from build123d import *

# Parameters (mm, degrees)
SKETCH1_R           = 1.5
BOSS_EXTRUDE1_DEPTH = 2
FILLET1_R           = 0.5
SKETCH3_R           = 2
SKETCH3_R_2         = 1.5
BOSS_EXTRUDE2_DEPTH = 0.5
BOSS_EXTRUDE2_TAPER = 5
FILLET2_R           = 0.1


with BuildPart() as part:
    # Sketch1 → Boss-Extrude1 (new body)
    with BuildSketch(Plane.XY):
        with BuildLine():
            Line((2.753751395, -0.013659805), (1.795799026, 2.087687523))
            ThreePointArc((1.795799026, 2.087687523), (1.631145222, 2.287378341), (1.388705435, 2.377988761))
            Line((1.388705435, 2.377988761), (-0.910090917, 2.599051338))
            ThreePointArc((-0.910090917, 2.599051338), (-1.165355141, 2.55630237), (-1.365045959, 2.391648566))
            Line((-1.365045959, 2.391648566), (-2.705889943, 0.511363815))
            ThreePointArc((-2.705889943, 0.511363815), (-2.796500362, 0.268924029), (-2.753751395, 0.013659805))
            Line((-2.753751395, 0.013659805), (-1.795799026, -2.087687523))
            ThreePointArc((-1.795799026, -2.087687523), (-1.631145222, -2.287378341), (-1.388705435, -2.377988761))
            Line((-1.388705435, -2.377988761), (0.910090917, -2.599051338))
            ThreePointArc((0.910090917, -2.599051338), (1.165355141, -2.55630237), (1.365045959, -2.391648566))
            Line((1.365045959, -2.391648566), (2.705889943, -0.511363815))
            ThreePointArc((2.705889943, -0.511363815), (2.796500362, -0.268924029), (2.753751395, -0.013659805))
        make_face()
        Circle(SKETCH1_R, mode=Mode.SUBTRACT)
    extrude(amount=BOSS_EXTRUDE1_DEPTH)

    # Fillet1
    fillet1_edges = [part.edges().sort_by_distance(p)[0] for p in [
        (1.165355141, -2.55630237, 2),
        (2.035467951, -1.45150619, 2),
        (2.796500362, -0.268924029, 2),
        (2.27477521, 1.037013859, 2),
        (1.631145222, 2.287378341, 2),
        (0.239307259, 2.488520049, 2),
        (-1.165355141, 2.55630237, 2),
        (-2.035467951, 1.45150619, 2),
        (-2.796500362, 0.268924029, 2),
        (-2.27477521, -1.037013859, 2),
        (-1.631145222, -2.287378341, 2),
        (-0.239307259, -2.488520049, 2),
    ]]
    fillet(fillet1_edges, radius=FILLET1_R)

    # Sketch3 → Boss-Extrude2 (add)
    with BuildSketch(Plane.XY.offset(2)):
        Circle(SKETCH3_R)
        Circle(SKETCH3_R_2, mode=Mode.SUBTRACT)
    extrude(amount=BOSS_EXTRUDE2_DEPTH, taper=BOSS_EXTRUDE2_TAPER)

    # Fillet2
    fillet2_edges = [part.edges().sort_by_distance(p)[0] for p in [
        (-2.27477521, -1.037013859, 0),
        (-2.796500362, 0.268924029, 0),
        (-2.035467951, 1.45150619, 0),
        (-1.165355141, 2.55630237, 0),
        (0.239307259, 2.488520049, 0),
        (1.631145222, 2.287378341, 0),
        (2.27477521, 1.037013859, 0),
        (2.796500362, -0.268924029, 0),
        (2.035467951, -1.45150619, 0),
        (1.165355141, -2.55630237, 0),
        (-0.239307259, -2.488520049, 0),
        (-1.631145222, -2.287378341, 0),
        (-1.956255668, 0, 2.5),
        (-1.543744332, 0, 2.5),
    ]]
    fillet(fillet2_edges, radius=FILLET2_R)


solid = part.part
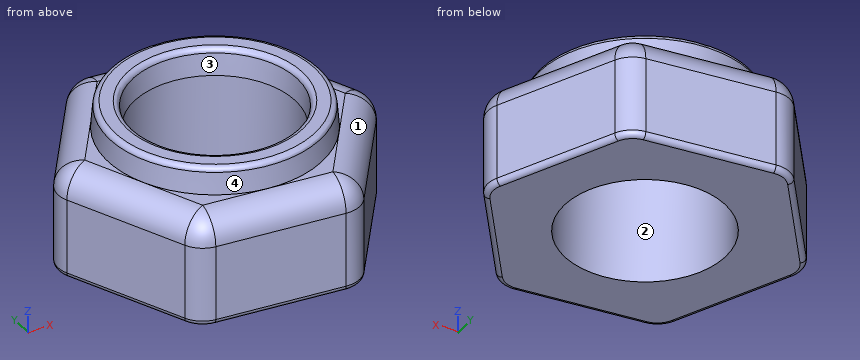
Input: part model. Units: mm. Frame: model coordinates. Face numbers are marked on the shaded views. Coordinates: 2 decimals unless noted, no trailing zeros. Loops run counter-clockwise (first coordinate to the right, second up) from the corner with the lowest first, then second, coordinate; pieces in that order, holes last.
Q1. Material intervals for line 1 (Z direction, x = -1.4, y = -1.75); line 2 (Y direction, x = 0.5, z = 2.35); line 3 (X direction, y = -0.6, z = 0.85), sorted ascending.
Q2. Cut plane A-A (z = 0.3). Output: boundary loops of the cut face in (x, y).
Q3. Draft query along Y for the marked faces 1, 2, 3 and 4. Return one class per face: +Y half, -Y half, draft (parallel to the pull), parting line (faces both ways), or undercut.
Q4. Cut plane B-B (z = 2.2). Output: boundary loops of the cut face in (x, y) (1 decimal).
Q5. Contact query for flat-ended pins moving along their axis: pin 1 (1 mm diameter, centred on x = -1, y = 2, fed in from +Z); pin 2 (1.5 mm diameter, centred on y = 1, z = 0.5, fed in from +X). Output: stop coordinate, or through.
Working result:
1. line 1: z = 0 to 2
1. line 2: y = -1.9 to -1.45, 1.45 to 1.9
1. line 3: x = -2.47 to -1.37, 1.37 to 2.64
2. outline: (-2.75, 0.01) - (-1.8, -2.09) arc R0.5 ccw to (-1.39, -2.38) - (0.91, -2.6) arc R0.5 ccw to (1.37, -2.39) - (2.71, -0.51) arc R0.5 ccw to (2.75, -0.01) - (1.8, 2.09) arc R0.5 ccw to (1.39, 2.38) - (-0.91, 2.6) arc R0.5 ccw to (-1.37, 2.39) - (-2.71, 0.51) arc R0.5 ccw to start; hole circle Ø3 at (0, 0)
3. face 1: -Y half
3. face 2: undercut
3. face 3: undercut
3. face 4: parting line
4. outline: circle Ø4 at (0, 0); hole circle Ø3 at (0, 0)
5. pin 1: stops at z = 2.5
5. pin 2: stops at x = 2.63
